Verification items for this drawing (mm, ordinates from the low corner). A direction names the side the tool comes from. Coordinates: 2 decimals unless noted, no trailing zeros. Order: outer loops, then holes, each group sorted by start corner. A loop starts at its lowest first (then second) coordinate and runs counter-clockwise, first axis right, second up. Notation, with made-up numbers: M 6,84 L 50,84 A28 cw 50,116 Z; hole C 48,55.25 d10. An arc over 180 degrees is marked long. Return JSON: item names as keys, results as strings. Group by question number.
1. Mould release check, pull along Z, two halves, no side actions. Record for the marked faces 1, 2 and 3: +Z half, -Z half, draft (parallel to the pull), parting line (faces both ways), or undercut.
2. Set-up check for the marked faces 4, 5 and 6: record each of +Z, -Z, +X, -X, +Y, -Y from which the full face is reachable in a straight line by a thin tool's end or side.
3. Gauge pin test, flat ends, axial feed: pin 1 (10.5 mm diameter, centred on y = 16.5, z = 90, fed in from +X); pin 2 (4 mm diameter, centred on x = 37, y = 42.5, fed in from -Z); pin 3 (2 mm diameter, centred on x = 27.5, z = 41.5, fed in from +Y); pin 4 (25 mm diameter, centred on y = 34.5, z = 18, fed in from -X). Record the tip position at first contact, or that the pin passes through.
4. Section check A-A, the plane y = 61.5. Record the cut outline in (x, z).
5. Material ranges on line 1 along Z through (x, y) = (64.5, 61.5); line 2 along Z through (x, y) = (16, 58); line 3 along X through (y, z) = (49.5, 25.5), recorded low to high.
6. Section check D-D, the plane y = 34.5. Record the cut outline in (x, z).
7. Section check C-C, the plane x = 28. Record the cut outline in (y, z), plus the area to 3 significant figures.
8. Section check B-B, the plane z = 14. Record the cut outline in (x, y), plus the area to 3 significant figures.
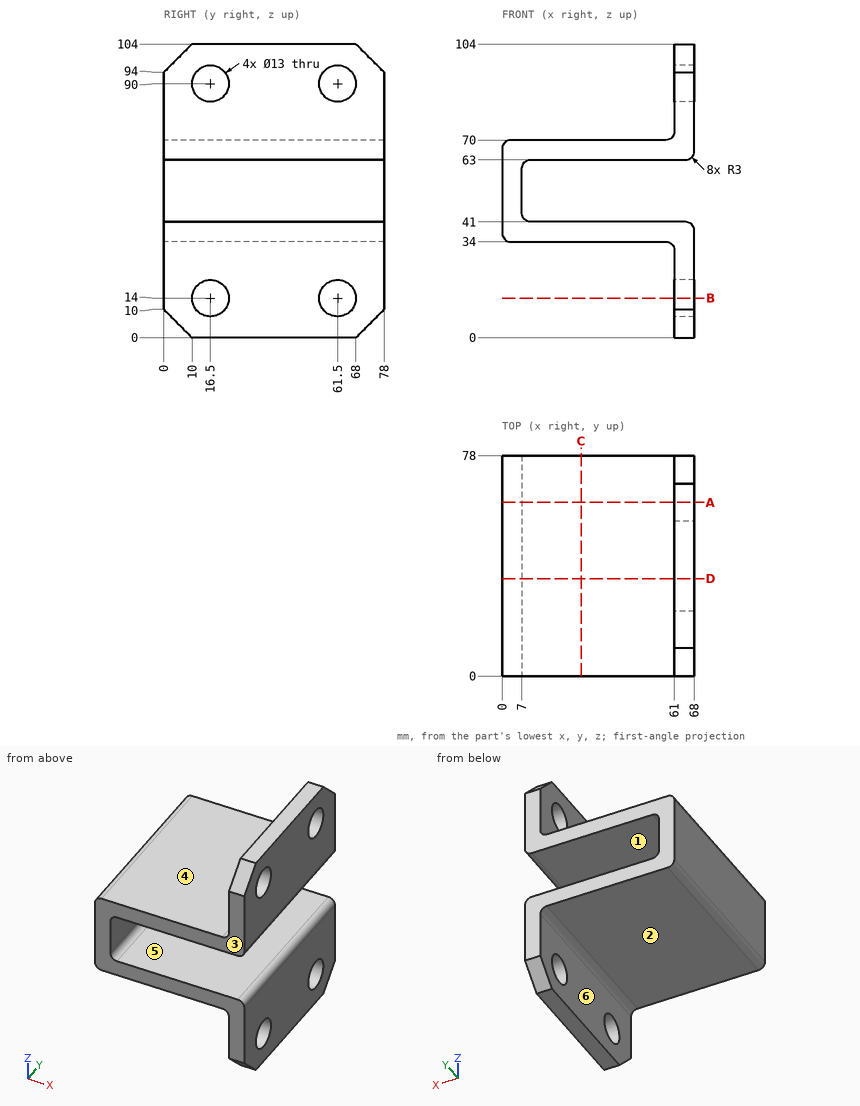
Answers follow:
{
 "1": {"face 1": "undercut", "face 2": "-Z half", "face 3": "draft"},
 "2": {"face 4": "+Z, -X, +Y, -Y", "face 5": "+X, +Y, -Y", "face 6": "-Z, -X, +Y, -Y"},
 "3": {"pin 1": "through", "pin 2": "z = 34", "pin 3": "y = 78", "pin 4": "x = 61"},
 "4": {"outline": "M 0,37 A3 ccw 3,34 L 58,34 A3 cw 61,31 L 61,20.5 L 68,20.5 L 68,38 A3 ccw 65,41 L 10,41 A3 cw 7,44 L 7,60 A3 cw 10,63 L 65,63 A3 ccw 68,66 L 68,83.5 L 61,83.5 L 61,73 A3 cw 58,70 L 3,70 A3 ccw 0,67 Z; M 61,0 L 68,0 L 68,7.5 L 61,7.5 Z; M 61,96.5 L 68,96.5 L 68,104 L 61,104 Z"},
 "5": {"line 1": "0 to 7.5, 20.5 to 41, 63 to 83.5, 96.5 to 104", "line 2": "34 to 41, 63 to 70", "line 3": "61 to 68"},
 "6": {"outline": "M 0,37 A3 ccw 3,34 L 58,34 A3 cw 61,31 L 61,0 L 68,0 L 68,38 A3 ccw 65,41 L 10,41 A3 cw 7,44 L 7,60 A3 cw 10,63 L 65,63 A3 ccw 68,66 L 68,104 L 61,104 L 61,73 A3 cw 58,70 L 3,70 A3 ccw 0,67 Z"},
 "7": {"outline": "M 0,34 L 78,34 L 78,41 L 0,41 Z; M 0,63 L 78,63 L 78,70 L 0,70 Z", "area": "1,090 mm^2"},
 "8": {"outline": "M 61,0 L 68,0 L 68,10 L 61,10 Z; M 61,23 L 68,23 L 68,55 L 61,55 Z; M 61,68 L 68,68 L 68,78 L 61,78 Z", "area": "364 mm^2"}
}
